Can you work these out from the drawing? Everything is in mm from the part's minimum corner. Coordinates: 2 decimals unless noted, no trailing zeros. Write each loop counter-clockwise with the first axis right and the second up, starting at its lowest first coordinate (ties: lowest second). Pieces come first, ordered by that corner, then holes. Notation, with made-up numbers: (82, -36) -> (98, -36) arc R28 ccw to (98, -12) -> close; hole circle Ø4 at (54.25, -33.75). An arc over 180 degrees is marked (long way). Use a Markdown table: item, result. Add a question column.
Item 1: Imagine slicing it at A-A, the plane z = 101.5. Write out the boundary of the cut face in (x, y).
Item 2: If I drill on line 1 along Z through (x, y) = (302, 15.75); line 2 along Z through (x, y) = (327, 8.5); line 3 along X through (y, z) = (10.75, 69.5), over which ranges is the centre line in solid material (lowest first)? Write a range as from..to.
Item 3: Imagine slicing it at B-B, the plane x = 251.5. Write out the boundary of the cut face in (y, z), and give its area (3 significant figures).
Item 4: Will this pin go through, and if not, where does the flat tip stop? pin 1 Ø3 at (x, y) = (311.5, 6) entering from -Z.
Item 5: Imagine slicing it at C-C, the plane y = 16.25. Write out the boundary of the cut face in (x, z), and give its area (3 significant figures).
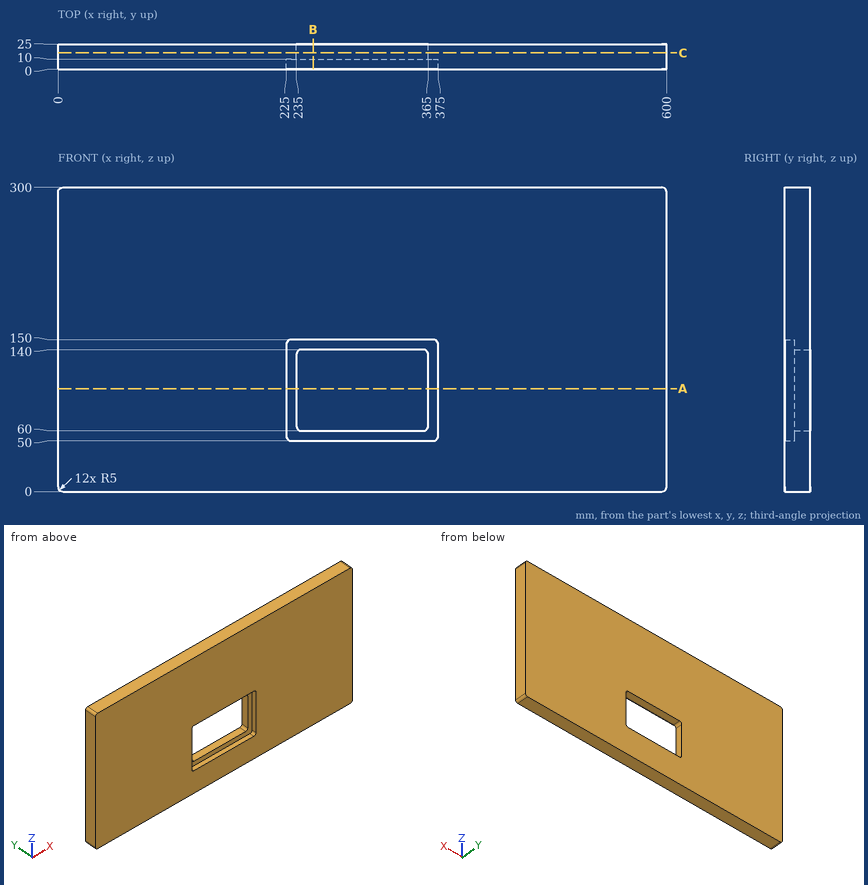
Ans:
| question | item | result |
|---|---|---|
| 1 | outline | (0, 0) -> (225, 0) -> (225, 10) -> (235, 10) -> (235, 25) -> (0, 25) -> close; (365, 10) -> (375, 10) -> (375, 0) -> (600, 0) -> (600, 25) -> (365, 25) -> close |
| 2 | line 1 | z = 0..60, 140..300 |
| 2 | line 2 | z = 0..50, 150..300 |
| 2 | line 3 | x = 0..235, 365..600 |
| 3 | outline | (0, 0) -> (25, 0) -> (25, 60) -> (10, 60) -> (10, 50) -> (0, 50) -> close; (0, 150) -> (10, 150) -> (10, 140) -> (25, 140) -> (25, 300) -> (0, 300) -> close |
| 3 | area | 5,300 mm^2 |
| 4 | pin 1 | stops at z = 0 |
| 5 | outline | (0, 5) arc R5 ccw to (5, 0) -> (595, 0) arc R5 ccw to (600, 5) -> (600, 295) arc R5 ccw to (595, 300) -> (5, 300) arc R5 ccw to (0, 295) -> close; hole (235, 65) arc R5 ccw to (240, 60) -> (360, 60) arc R5 ccw to (365, 65) -> (365, 135) arc R5 ccw to (360, 140) -> (240, 140) arc R5 ccw to (235, 135) -> close |
| 5 | area | 170,000 mm^2 |
